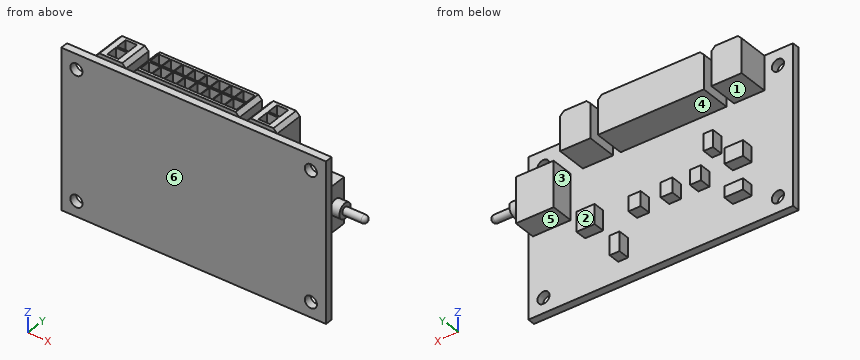
```python
from build123d import *

# Parameters (mm, degrees)
SKETCH1_W           = 70
SKETCH1_H           = 42
BOSS_EXTRUDE1_DEPTH = 2
SKETCH4_R           = 1.6
CUT_EXTRUDE2_DEPTH  = 82.65782265
BOSS_EXTRUDE2_DEPTH = 8
SKETCH6_W           = 3
SKETCH6_H           = 3
CUT_EXTRUDE3_DEPTH  = 9
SKETCH7_W           = 10
SKETCH7_H           = 12
BOSS_EXTRUDE3_DEPTH = 6
SKETCH8_R           = 2
BOSS_EXTRUDE4_DEPTH = 2.5
SKETCH9_R           = 1
BOSS_EXTRUDE5_DEPTH = 5
SKETCH10_W          = 4.972668361
SKETCH10_H          = 2.900723211
SKETCH10_H_2        = 4.06167287
SKETCH10_W_2        = 4.792773987
SKETCH10_H_3        = 5.198941274
SKETCH10_W_3        = 2.924404467
SKETCH10_H_4        = 3.899205956
SKETCH10_W_4        = 3.086871382
SKETCH10_W_5        = 3.249338296
SKETCH10_W_6        = 2.437003722
SKETCH10_H_5        = 4.467840158
SKETCH10_W_7        = 2.599470637
SKETCH10_H_6        = 5.088357614
BOSS_EXTRUDE6_DEPTH = 3


# Read off the part's stored shape, not the designer's step: Dome1
with BuildPart() as part:
    # Sketch1 → Boss-Extrude1 (new body)
    with BuildSketch(Plane(origin=(0, 0, 0), x_dir=(1, 0, 0), z_dir=(0, 1, 0))):
        with Locations((35, 21)):
            Rectangle(SKETCH1_W, SKETCH1_H)
    extrude(amount=BOSS_EXTRUDE1_DEPTH)

    # Sketch4 → Cut-Extrude2 (cut, through all)
    with BuildSketch(Plane(origin=(0, 2, 0), x_dir=(1, 0, 0), z_dir=(0, 1, 0))):
        with Locations(Location((4, 38, 0), (0, 0, 270))):
            Circle(SKETCH4_R)
        with Locations(Location((66, 4, 0), (0, 0, 270))):
            Circle(SKETCH4_R)
        with Locations(Location((4, 4, 0), (0, 0, 90))):
            Circle(SKETCH4_R)
        with Locations(Location((66, 38, 0), (0, 0, 90))):
            Circle(SKETCH4_R)
    extrude(amount=-CUT_EXTRUDE2_DEPTH, mode=Mode.SUBTRACT)

    # Sketch5 → Boss-Extrude2 (add)
    with BuildSketch(Plane(origin=(0, 2, 0), x_dir=(1, 0, 0), z_dir=(0, 1, 0))):
        Polygon((17.6, 9), (45.6, 9), (45.6, 0), (44.6, -1), (18.6, -1), (17.6, 0), align=None)
        Polygon((7.6, 9), (15.6, 9), (15.6, 0), (14.6, -1), (8.6, -1), (7.6, 0), align=None)
        Polygon((47.6, 9), (55.6, 9), (55.6, 0), (54.6, -1), (48.6, -1), (47.6, 0), align=None)
    extrude(amount=BOSS_EXTRUDE2_DEPTH)

    # Sketch6 → Cut-Extrude3 (cut)
    with BuildSketch(Plane.XY.offset(1)):
        with Locations((20.35, 4.25)):
            Rectangle(SKETCH6_W, SKETCH6_H)
        with Locations((11.6, 7.75)):
            Rectangle(SKETCH6_W, SKETCH6_H)
        with Locations((23.55, 4.25)):
            Rectangle(SKETCH6_W, SKETCH6_H)
        with Locations((11.6, 4.25)):
            Rectangle(SKETCH6_W, SKETCH6_H)
        with Locations((20.35, 7.75)):
            Rectangle(SKETCH6_W, SKETCH6_H)
        with Locations((51.6, 7.75)):
            Rectangle(SKETCH6_W, SKETCH6_H)
        with Locations((23.55, 7.75)):
            Rectangle(SKETCH6_W, SKETCH6_H)
        with Locations((26.75, 4.25)):
            Rectangle(SKETCH6_W, SKETCH6_H)
        with Locations((26.75, 7.75)):
            Rectangle(SKETCH6_W, SKETCH6_H)
        with Locations((29.95, 4.25)):
            Rectangle(SKETCH6_W, SKETCH6_H)
        with Locations((29.95, 7.75)):
            Rectangle(SKETCH6_W, SKETCH6_H)
        with Locations((33.15, 4.25)):
            Rectangle(SKETCH6_W, SKETCH6_H)
        with Locations((33.15, 7.75)):
            Rectangle(SKETCH6_W, SKETCH6_H)
        with Locations((36.35, 4.25)):
            Rectangle(SKETCH6_W, SKETCH6_H)
        with Locations((36.35, 7.75)):
            Rectangle(SKETCH6_W, SKETCH6_H)
        with Locations((39.55, 4.25)):
            Rectangle(SKETCH6_W, SKETCH6_H)
        with Locations((39.55, 7.75)):
            Rectangle(SKETCH6_W, SKETCH6_H)
        with Locations((42.75, 4.25)):
            Rectangle(SKETCH6_W, SKETCH6_H)
        with Locations((42.75, 7.75)):
            Rectangle(SKETCH6_W, SKETCH6_H)
        with Locations((51.6, 4.25)):
            Rectangle(SKETCH6_W, SKETCH6_H)
    extrude(amount=-CUT_EXTRUDE3_DEPTH, mode=Mode.SUBTRACT)

    # Sketch7 → Boss-Extrude3 (add)
    with BuildSketch(Plane(origin=(0, 2, 0), x_dir=(1, 0, 0), z_dir=(0, 1, 0))):
        with Locations((63.8, 15)):
            Rectangle(SKETCH7_W, SKETCH7_H)
    extrude(amount=BOSS_EXTRUDE3_DEPTH)

    # Sketch8 → Boss-Extrude4 (add)
    with BuildSketch(Plane(origin=(68.8, 0, 0), x_dir=(0, 0, -1), z_dir=(1, 0, 0))):
        with Locations(Location((15, 5, 0), (0, 0, 180))):
            Circle(SKETCH8_R)
    extrude(amount=BOSS_EXTRUDE4_DEPTH)

    # Sketch9 → Boss-Extrude5 (add)
    with BuildSketch(Plane(origin=(71.3, 0, 0), x_dir=(0, 0, -1), z_dir=(1, 0, 0))):
        with Locations((15, 5)):
            Circle(SKETCH9_R)
    extrude(amount=BOSS_EXTRUDE5_DEPTH)

    # Dome1 outline → Dome1 (revolve)
    with BuildSketch(Plane(origin=(0, 5, -15), x_dir=(0, 1, 0), z_dir=(0, 0, -1))):
        with BuildLine():
            Line((0, 76.3), (1, 76.299999999))
            ThreePointArc((1, 76.299999999), (0.707106782, 77.007106781), (0, 77.3))
            Line((0, 77.3), (0, 76.3))
        make_face()
    revolve(axis=Axis((0, 5, -15), (1, 0, 0)))

    # Sketch10 → Boss-Extrude6 (add)
    with BuildSketch(Plane(origin=(0, 2, 0), x_dir=(1, 0, 0), z_dir=(0, 1, 0))):
        with Locations((13.43956041, 33.400988797)):
            Rectangle(SKETCH10_W, SKETCH10_H)
        with Locations((13.43956041, 24.122865076)):
            Rectangle(SKETCH10_W, SKETCH10_H_2)
        with Locations((52.609554771, 24.691499278)):
            Rectangle(SKETCH10_W_2, SKETCH10_H_3)
        with Locations((23.568593744, 25.828767682)):
            Rectangle(SKETCH10_W_3, SKETCH10_H_4)
        with Locations((31.204538742, 25.828767682)):
            Rectangle(SKETCH10_W_4, SKETCH10_H_4)
        with Locations((39.652818313, 25.828767682)):
            Rectangle(SKETCH10_W_5, SKETCH10_H_4)
        with Locations((20.156788533, 18.314672871)):
            Rectangle(SKETCH10_W_6, SKETCH10_H_5)
        with Locations((44.932993045, 34.494805998)):
            Rectangle(SKETCH10_W_7, SKETCH10_H_6)
    extrude(amount=BOSS_EXTRUDE6_DEPTH)


solid = part.part
```
Check sheet for the modelled part. Datum: model origin and axes. Units: mm. Face numbers are marked on the shaded views. A direction names the side the tool comes from. Round coordinates to 2 decimals unless told otherwise and drop trailing zeros. Write each loop counter-clockwise with the first axis right and the second up, starting at its lowest first coordinate (ties: lowest second). Pieces come first, ordered by that corner, then holes. Notation, with made-up numbers: (51.5, -24) -> (74.5, -24) arc R19 ccw to (74.5, -11) -> close; hole circle Ø8 at (-23.75, -27.75). An arc over 180 degrees is marked (long way). Put each result on its own line as item: value.
(1) Sectioned sample at B-B (x = 4). Enter the section's corners in (y, z), plus the area to 3 significant figures.
Values found:
outline: (0, -42) -> (2, -42) -> (2, -39.6) -> (0, -39.6) -> close; (0, -36.4) -> (2, -36.4) -> (2, -5.6) -> (0, -5.6) -> close; (0, -2.4) -> (2, -2.4) -> (2, 0) -> (0, 0) -> close
area: 71.2 mm^2
(2) Sectioned sample at D-D (z = -4). Count the separate pieces of the cut face and the enclosed holes in it, plus the area to 3 significant figures.
Values found:
separate pieces: 3
enclosed holes: 20
area: 299 mm^2
(3) Tool access check on the marked faces 1, 2 and 3. Record the directions out of +Z, -Z, +X, -X, +Y, -Y that give a thin tool (end or side, any length) a straight path to the whole face; none if there is none.
Values found:
face 1: -X, +Y
face 2: -Z, +X, -X, +Y
face 3: +Z, -Z, +Y
(4) Mould release check, pull along Z, two halves, no side actions. Record for the marked faces 4, 5 and 6: released by +Z, released by -Z, zero draft, split by the parting line, or undercut.
Values found:
face 4: undercut
face 5: released by -Z
face 6: zero draft
(5) Go/stop test with flat-tipped pins: pin 1 Ø1.5 at (x, z) = (49.5, -10) entering from -Y; pin 2 Ø5 at (x, z) = (64, -25.5) entering from +Y; pin 3 Ø1.8 at (y, z) = (5, -14) entering from -X; pin 4 Ø1.5 at (y, z) = (4.5, -28) entering from -X. Record where each tip stops, or that it passes through.
Values found:
pin 1: stops at y = 0
pin 2: stops at y = 2
pin 3: stops at x = 58.8
pin 4: stops at x = 22.11
(6) Material ranges on line 1 (Y direction, x = 25.5, z = -5.5); line 2 (X direction, y = 4, z = -8.5); line 3 (X direction, y = 0.8, z = -38), recorded low to high.
Values found:
line 1: y = 0 to 2.75, 5.75 to 6.25, 9.25 to 10
line 2: x = 7.6 to 15.6, 17.6 to 45.6, 47.6 to 55.6
line 3: x = 0 to 2.4, 5.6 to 64.4, 67.6 to 70
(7) Sectioned sample at A-A (z = -38). Enter the section's corners in (x, y).
Values found:
outline: (0, 0) -> (2.4, 0) -> (2.4, 2) -> (0, 2) -> close; (5.6, 0) -> (64.4, 0) -> (64.4, 2) -> (5.6, 2) -> close; (67.6, 0) -> (70, 0) -> (70, 2) -> (67.6, 2) -> close
(8) Sectioned sample at C-C (x = 24). Enter the section's corners in (y, z), plus the area to 3 significant figures.
Values found:
outline: (0, -42) -> (2, -42) -> (2, -27.78) -> (5, -27.78) -> (5, -23.88) -> (2, -23.88) -> (2, -9) -> (10, -9) -> (10, 1) -> (9.25, 1) -> (9.25, -8) -> (6.25, -8) -> (6.25, 1) -> (5.75, 1) -> (5.75, -8) -> (2.75, -8) -> (2.75, 1) -> (2, 1) -> (2, 0) -> (0, 0) -> close
area: 122 mm^2
